from build123d import *

# Parameters (mm, degrees)
SKETCH1_R           = 5
SKETCH1_R_2         = 3.175
BOSS_EXTRUDE1_DEPTH = 15
SKETCH2_W           = 9
SKETCH2_H           = 1


with BuildPart() as part:
    # Sketch1 → Boss-Extrude1 (new body)
    with BuildSketch(Plane(origin=(0, 0, 0), x_dir=(0, 0, -1), z_dir=(1, 0, 0))):
        Circle(SKETCH1_R)
        Circle(SKETCH1_R_2, mode=Mode.SUBTRACT)
    extrude(amount=BOSS_EXTRUDE1_DEPTH)

    # Sketch2 → Cut-Revolve1 (revolve, cut)
    with BuildSketch(Plane.XY, mode=Mode.PRIVATE) as cut_revolve1_sk:
        with Locations((7.5, 4.5)):
            Rectangle(SKETCH2_W, SKETCH2_H)
    revolve(cut_revolve1_sk.sketch.rotate(Axis((15, 0, 0), (-1, 0, 0)), 90), axis=Axis((15, 0, 0), (-1, 0, 0)), mode=Mode.SUBTRACT)

    # Sketch3 → #60 (0.04) Diameter Hole1 (revolve, cut)
    with BuildSketch(Plane.YZ.offset(1.382942836)):
        Polygon((0, 0), (0, 25.705237194), (0.508, 25.4), (0.508, 0), align=None)
    revolve(axis=Axis((1.382942836, 0, -6.35), (0, 0, 1)), mode=Mode.SUBTRACT)


solid = part.part
Build history of the part. All positions in model axes, mm. A direction names the side the tool comes from. Round coordinates to 2 decimals unless told otherwise and drop trailing zeros. Write each loop counter-clockwise with the first axis right and the second up, starting at its lowest first coordinate (ties: lowest second). Pieces come first, ordered by that corner, then holes. Notation, with made-up numbers: M -21,26 L -2,26 A29 cw -2,49 Z; hole C -21.5,19.5 d8. An arc over 180 degrees is marked long. Answer as a JSON object with one key per item and string values. Group by question number.
(1) Mould opens along X. For faces 1 (the flat face through (15, -3.3, -1)), 2 (the cylindrical face through (1.88, -0.11, 4.05)), 3 (the flat face through (0, -3.3, -1)) say: pulls with the +X half, pulls with the -X half, needs draft (parallel to the pull), parting line crosses it, or undercut.
(2) Which spindle directions (+Z, -Z, +X, -X, +Y, -Y) get a long thin tool onto all of the face, cutting with end or side? Do faces 4 (the cylindrical face through (7.563, 3.905, 0.867)), 5 (the cylindrical face through (7.4, -3.1, 0.69)). Say none if no direction does.
(3) Cut at A-A (y = 0). Give the cut face in (x, z) (3 decimals).
(4) Cut at B-B (z = 0). Give the cut face in (x, y) (3 decimals).
(5) Cut at D-D (x = 6.5). Give the cut face in (y, z) (3 decimals), and give its area (3 significant figures).
(6) Drill centre lines: L1, parallel to X at y = -3.25, z = 2.5; L2, parallel to Z at x = 8.25, y = 0.75; L3, parallel to Z at x = 9.75, y = -1. Where is each one in solid material? Low to high.
(7) Flat gauge pins, fed straight in: pin 1 (2 mm diameter, centred on x = 8, z = 2, fed in from -Y); pin 2 (1 mm diameter, centred on y = -2, z = 1.5, fed in from -X); pin 3 (6 mm diameter, centred on x = 11, z = -4, fed in from +Y). Where does each tip first touch, or does it go through?
(8) Cut at C-C (y = -2.5). Give the cut face in (x, z).
Responses:
{
 "1": {"face 1": "pulls with the +X half", "face 2": "undercut", "face 3": "pulls with the -X half"},
 "2": {"face 4": "none", "face 5": "+X, -X"},
 "3": {"outline": "M 0,-5 L 3,-5 L 3,-4 L 12,-4 L 12,-5 L 15,-5 L 15,-3.175 L 0,-3.175 Z; M 0,3.175 L 0.875,3.175 L 0.875,5 L 0,5 Z; M 1.891,3.175 L 15,3.175 L 15,5 L 12,5 L 12,4 L 3,4 L 3,5 L 1.891,5 Z"},
 "4": {"outline": "M 0,-5 L 3,-5 L 3,-4 L 12,-4 L 12,-5 L 15,-5 L 15,-3.175 L 0,-3.175 Z; M 0,3.175 L 15,3.175 L 15,5 L 12,5 L 12,4 L 3,4 L 3,5 L 0,5 Z"},
 "5": {"outline": "C 0,0 d8; hole C 0,0 d6.35", "area": "18.6 mm2"},
 "6": {"L1": "x = 0 to 3, 12 to 15", "L2": "z = -3.93 to -3.09, 3.09 to 3.93", "L3": "z = -3.87 to -3.01, 3.01 to 3.87"},
 "7": {"pin 1": "stops at y = -3.87", "pin 2": "passes through", "pin 3": "stops at y = 4.86"},
 "8": {"outline": "M 0,-4.33 L 3,-4.33 L 3,-3.12 L 12,-3.12 L 12,-4.33 L 15,-4.33 L 15,-1.96 L 0,-1.96 Z; M 0,1.96 L 15,1.96 L 15,4.33 L 12,4.33 L 12,3.12 L 3,3.12 L 3,4.33 L 0,4.33 Z"}
}
